```python
from build123d import *

# Parameters (mm, degrees)
F0_W     = 27.375
F0_H     = 25
F0_W_2   = 20
F0_H_2   = 55
F1_DEPTH = 5
F2_W     = 5
F2_H     = 25
F2_H_2   = 5
F3_DEPTH = 17.5
F4_W     = 25
F4_H     = 2.5
F5_DEPTH = 3
F6_W     = 25
F6_H     = 2.5
F7_DEPTH = 3
F8_R     = 1


with BuildPart() as f1:
    # F0 (on Top) → F1 (new body)
    with BuildSketch(Plane.XY):
        with Locations((-23.6875, 0)):
            Rectangle(F0_W, F0_H)
        Rectangle(F0_W_2, F0_H)
        with Locations((23.6875, 0)):
            Rectangle(F0_W, F0_H)
        with Locations((0, -40)):
            Rectangle(F0_W_2, F0_H_2)
    extrude(amount=F1_DEPTH)

    # F2 (on Top) → F3 (join)
    with BuildSketch(Plane.XY):
        with Locations((-39.875, 0)):
            Rectangle(F2_W, F2_H)
        with Locations((39.875, 0)):
            Rectangle(F2_W, F2_H)
        with Locations((-7.5, -70)):
            Rectangle(F2_W, F2_H_2)
        with Locations((7.5, -70)):
            Rectangle(F2_W, F2_H_2)
    extrude(amount=F3_DEPTH)

    # F4 (on face) → F5 (join)
    with BuildSketch(Plane.YZ.offset(-37.375)):
        with Locations((0, 16.25)):
            Rectangle(F4_W, F4_H)
    extrude(amount=F5_DEPTH)

    # F6 (on face) → F7 (join)
    with BuildSketch(Plane(origin=(37.375, 0, 0), x_dir=(0, -1, 0), z_dir=(-1, 0, 0))):
        with Locations((0, 16.25)):
            Rectangle(F6_W, F6_H)
    extrude(amount=F7_DEPTH)

    # F8
    f8_edges = [f1.edges().sort_by_distance(p)[0] for p in [
        (-37.375, 0, 5),
        (37.375, 0, 5),
        (7.5, -67.5, 17.5),
        (-7.5, -67.5, 17.5),
        (7.5, -67.5, 5),
        (-7.5, -67.5, 5),
        (-42.375, -12.5, 8.75),
        (-42.375, 12.5, 8.75),
        (-42.375, 0, 17.5),
        (42.375, 0, 17.5),
        (42.375, -12.5, 8.75),
        (42.375, 12.5, 8.75),
        (-10, -72.5, 8.75),
        (10, -72.5, 8.75),
        (-34.375, 0, 17.5),
        (-34.375, 0, 15),
        (34.375, 0, 17.5),
        (34.375, 0, 15),
        (37.375, 0, 15),
        (-37.375, 0, 15),
    ]]
    fillet(f8_edges, radius=F8_R)


solid = f1.part
```
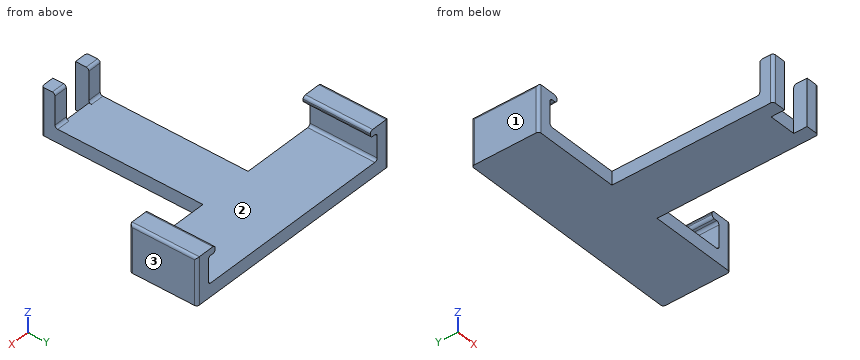
Source: CAD feature listing. Evaluate the final solid. Frame: model axes, mm. Face numbers are marked on the shaded views. Coordinates: 2 decimals unless noted, no trailing zeros. Order: outer loops, then holes, each group sorted by start corner. A loop starts at its lowest first (then second) coordinate and runs counter-clockwise, first axis right, second up. Notation, with made-up numbers: (13.25, -38.5) - (28.25, -38.5) arc R20 cw to (28.25, -30.5) - close; hole circle Ø3 at (71.25, 4). An arc over 180 degrees is marked (long way). One line per item, written item: value.
1) Mould query, pull axis X, two halves, no side actions, for the marked faces 1, 2 and 3. Classes: released by +X, released by -X, zero draft, split by the parting line, or undercut.
Computed values:
face 1: released by -X
face 2: undercut
face 3: released by +X
2) Cut plane D-D on y = -22. Output: boundary loops of the cut face in (x, z).
Computed values:
outline: (-10, 0) - (10, 0) - (10, 5) - (-10, 5) - close
3) Contact query for flat-ended pins moving along their axis: pin 1 (5 mm diameter, centred on y = -68.5, z = 6, fed in from +X); pin 2 (5.5 mm diameter, centred on x = 2, z = 3.5, fed in from -Y); pin 3 (5 mm diameter, centred on y = -70, z = 11, fed in from -X); pin 4 (5 mm diameter, centred on x = -32.5, z = 9.5, fed in from -Y). Output: stop coordinate, or through.
Computed values:
pin 1: stops at x = 10
pin 2: stops at y = -67.5
pin 3: stops at x = -10
pin 4: passes through
4) Cut plane B-B on y = -8.5. Output: boundary loops of the cut face in (x, z) (3 decimals), plus the area to 3 significant figures.
Computed values:
outline: (-42.375, 0) - (42.375, 0) - (42.375, 16.5) arc R1 ccw to (41.375, 17.5) - (35.375, 17.5) arc R1 ccw to (34.375, 16.5) - (34.375, 16) arc R1 ccw to (35.375, 15) - (36.375, 15) arc R1 cw to (37.375, 14) - (37.375, 6) arc R1 cw to (36.375, 5) - (-36.375, 5) arc R1 cw to (-37.375, 6) - (-37.375, 14) arc R1 cw to (-36.375, 15) - (-35.375, 15) arc R1 ccw to (-34.375, 16) - (-34.375, 16.5) arc R1 ccw to (-35.375, 17.5) - (-41.375, 17.5) arc R1 ccw to (-42.375, 16.5) - close
area: 563 mm^2
5) Cut plane A-A on z = 9.5. Output: boundary loops of the cut face in (x, y) (3 decimals).
Computed values:
outline: (-42.375, -11.5) arc R1 ccw to (-41.375, -12.5) - (-37.375, -12.5) - (-37.375, 12.5) - (-41.375, 12.5) arc R1 ccw to (-42.375, 11.5) - close; (-10, -71.5) arc R1 ccw to (-9, -72.5) - (-5, -72.5) - (-5, -67.5) - (-10, -67.5) - close; (5, -72.5) - (9, -72.5) arc R1 ccw to (10, -71.5) - (10, -67.5) - (5, -67.5) - close; (37.375, -12.5) - (41.375, -12.5) arc R1 ccw to (42.375, -11.5) - (42.375, 11.5) arc R1 ccw to (41.375, 12.5) - (37.375, 12.5) - close
6) Ray query, line 1 (X direction, y = -8, z = 10.5) (3 decimals); line 2 (X direction, y = -68, z = 10.25); line 3 (Z direction, x = 7.5, y = -40). Return the intervals inside material, ascending. Write a range as [from, to].
Computed values:
line 1: x = [-42.375, -37.375], [37.375, 42.375]
line 2: x = [-10, -5], [5, 10]
line 3: z = [0, 5]
7) Cut plane C-C on x = -29. Output: boundary loops of the cut face in (y, z).
Computed values:
outline: (-12.5, 0) - (12.5, 0) - (12.5, 5) - (-12.5, 5) - close
